Source: CAD feature listing. Evaluate the final solid. Frame: model axes, mm. A direction names the side the tool comes from. Round coordinates to 2 decimals unless told otherwise and drop trailing zeros. Order: outer loops, then holes, each group sorted by start corner. A loop starts at its lowest first (then second) coordinate and runs counter-clockwise, first axis right, second up. Notation, with made-up numbers: (13.25, 71.25) -> (24.25, 71.25) arc R14 cw to (24.25, 77.25) -> close; hole circle Ø5 at (70.25, -21). An arc over 180 degrees is marked (long way). Write item = value, one per line. Start each with the question number.
(1) Cut plane C-C on x = 12. Return the cut outline in (y, z).
(2) Draft query along Y for faces 5 (the face through (0, -12, 3)), 6 (the face through (2.13, 6.24, 2.46)), 7 (the face through (-15, -3, 3)). Return one class per face: released by +Y, released by -Y, zero draft, split by the parting line, or undercut.
(3) Ray query, line 1 (X direction, y = -10.95, z = -2.5); line 2 (Z direction, x = -12.25, y = -11); line 3 (X direction, y = -10.5, z = -1.75). Return the intervals inside material, ascending.
(4) Cut plane A-A on y = 0. Return the cut outline in (x, z).
(5) Contact query for flat-ended pins moving along their axis: pin 1 Ø4 at (x, y) = (-11, 2.5) entering from -Z; pin 2 Ø3 at (x, z) = (4.5, 8) entering from +Y. Output: stop coordinate, or through.
(6) Cut plane B-B on z = 7.5. Return the cut outline in (x, y).
(7) Cut plane D-D on z = 3.5. Return the cut outline in (x, y).
(8) Reachability of faces 1 (the face through (0, -10, 8)), 2 (the face through (0, -10, -3)), 3 (the face through (-13.513, -10.986, 7.164)), 4 (the face through (-2.21, 6.14, 2.46)) from +Z, -Z, +X, -X, +Y, -Y: full face, straight path, thin tool, end or side. Return the list, or none.
from build123d import *

# Parameters (mm, degrees)
EXTRUDE_1_DEPTH     = 5
SKETCH_2_W          = 15
SKETCH_2_H          = 5
EXTRUDE_3_DEPTH     = 2
SKETCH_4_R          = 1.55
CUT_EXTRUDE_1_DEPTH = 2
SKETCH_7_R          = 5.5
CUT_EXTRUDE_7_DEPTH = 10


with BuildPart() as part:
    # 草图1 → 凸台-拉伸1 (new body)
    with BuildSketch(Plane.XY):
        Polygon((15, 10), (0, 10), (-15, 10), (-15, -10), (15, -10), align=None)
        with BuildLine():
            Line((-4.044639437, 3.577833398), (0, 8.150214535))
            Line((0, 8.150214535), (4.04465135, 3.577819931))
            ThreePointArc((4.04465135, 3.577819931), (5.049807783, 1.912966637), (5.4, 0))
            ThreePointArc((5.4, 0), (-1.912975044, -5.049804598), (-4.044639437, 3.577833398))
        make_face(mode=Mode.SUBTRACT)
    extrude(amount=EXTRUDE_1_DEPTH)

    # 草图2 → 凸台-拉伸3 (add)
    with BuildSketch(Plane.XZ.offset(10)):
        Polygon((15, 0), (0, 0), (-15, 0), (-15, -5.5), (15, -5.5), align=None)
        Polygon((-15, 5), (0, 5), (15, 5), (15, 10.5), (-15, 10.5), align=None)
        with Locations((-7.5, 2.5)):
            Rectangle(SKETCH_2_W, SKETCH_2_H)
        with Locations((7.5, 2.5)):
            Rectangle(SKETCH_2_W, SKETCH_2_H)
    extrude(amount=EXTRUDE_3_DEPTH)

    # 草图4 → 切除-拉伸1 (cut)
    with BuildSketch(Plane(origin=(0, -10, 0), x_dir=(1, 0, 0), z_dir=(0, 1, 0))):
        with BuildLine():
            ThreePointArc((-10.45, 2.5), (-10.903984489, 3.596015511), (-12, 4.05))
            Line((-12, 4.05), (-12, 2.5))
            Line((-12, 2.5), (-13.55, 2.5))
            ThreePointArc((-13.55, 2.5), (-12, 0.95), (-10.45, 2.5))
        make_face()
        with BuildLine():
            Line((-12, 2.5), (-12, 4.05))
            ThreePointArc((-12, 4.05), (-13.096015511, 3.596015511), (-13.55, 2.5))
            Line((-13.55, 2.5), (-12, 2.5))
        make_face()
        with Locations(Location((12, 2.5, 0), (0, 0, 270))):
            Circle(SKETCH_4_R)
        with Locations(Location((12, -7.5, 0), (0, 0, 270))):
            Circle(SKETCH_4_R)
        with Locations(Location((-12, -7.5, 0), (0, 0, 270))):
            Circle(SKETCH_4_R)
    extrude(amount=-CUT_EXTRUDE_1_DEPTH, mode=Mode.SUBTRACT)

    # 草图7 → 切除-拉伸7 (cut)
    with BuildSketch(Plane(origin=(0, 0, 0), x_dir=(-1, 0, 0), z_dir=(0, 0, -1))):
        with BuildLine():
            Line((-3.352919189, 4.359808816), (0, 8.150214535))
            Line((0, 8.150214535), (0, 9))
            Line((0, 9), (-4.326606057, 3.395656052))
            ThreePointArc((-4.326606057, 3.395656052), (-3.869906283, 3.908174172), (-3.352919189, 4.359808816))
        make_face()
        with BuildLine():
            Line((0, 9), (0, 8.150214535))
            Line((0, 8.150214535), (3.352919189, 4.359808816))
            ThreePointArc((3.352919189, 4.359808816), (3.885429206, 3.89274195), (4.353496537, 3.361111111))
            Line((4.353496537, 3.361111111), (0, 9))
        make_face()
        Circle(SKETCH_7_R)
        with BuildLine():
            Line((0, 8.150214535), (4.044639437, 3.577833398))
            ThreePointArc((4.044639437, 3.577833398), (8.99e-06, -5.4), (-4.04465135, 3.577819931))
            Line((-4.04465135, 3.577819931), (0, 8.150214535))
        make_face()
    extrude(amount=-CUT_EXTRUDE_7_DEPTH, mode=Mode.SUBTRACT)


solid = part.part
Evaluation:
q1.outline = (-12, -5.5) -> (-10, -5.5) -> (-10, -4.05) -> (-12, -4.05) -> close; (-12, -0.95) -> (-10, -0.95) -> (-10, 0) -> (10, 0) -> (10, 5) -> (-10, 5) -> (-10, 5.95) -> (-12, 5.95) -> close; (-12, 9.05) -> (-10, 9.05) -> (-10, 10.5) -> (-12, 10.5) -> close
q2.face_5 = released by -Y
q2.face_6 = undercut
q2.face_7 = zero draft
q3.line_1 = -15 to -13.55, -10.45 to 10.45, 13.55 to 15
q3.line_2 = -5.5 to -4.03, -0.97 to 5.97, 9.03 to 10.5
q3.line_3 = -15 to -13.36, -10.64 to 10.64, 13.36 to 15
q4.outline = (-15, 0) -> (-5.5, 0) -> (-5.5, 5) -> (-15, 5) -> close; (5.5, 0) -> (15, 0) -> (15, 5) -> (5.5, 5) -> close
q5.pin_1 = 0
q5.pin_2 = -10
q6.outline = (-15, -12) -> (-13.55, -12) -> (-13.55, -10) -> (-15, -10) -> close; (-10.45, -12) -> (10.45, -12) -> (10.45, -10) -> (-10.45, -10) -> close; (13.55, -12) -> (15, -12) -> (15, -10) -> (13.55, -10) -> close
q7.outline = (-15, -12) -> (15, -12) -> (15, 10) -> (-15, 10) -> close; hole (-4.35, 3.36) arc R5.5 ccw (long way) to (4.33, 3.4) -> (0, 9) -> close
q8.face_1 = +Z, +X, -X, +Y
q8.face_2 = -Z, +X, -X, +Y
q8.face_3 = +Y, -Y
q8.face_4 = +Z, -Z
